Check sheet for the modelled part. Datum: model origin and axes. Units: mm. Coordinates: 2 decimals unless noted, no trailing zeros. Loops run counter-clockwise (first coordinate to the right, second up) from the corner with the lowest first, then second, coordinate; pieces in that order, holes last. Notation, with made-up numbers: (-15.5, 38) -> (0.5, 38) arc R21 cw to (0.5, 57) -> close; hole circle Ø8 at (38, 59). An arc over 180 degrees is marked (long way). Use one line per item in the form item = value.
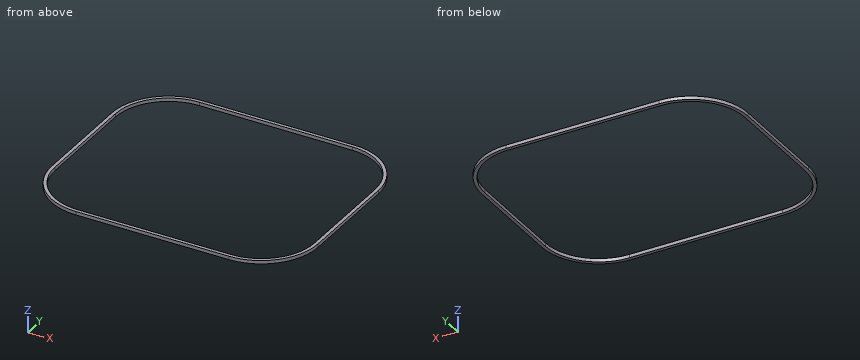
from build123d import *

# Parameters (mm, degrees)
F0_W     = 500
F0_H     = 6.35
F1_DEPTH = 410
F3_DEPTH = 25
F4_W     = 517.022076
F4_H     = 424.169128
F5_DEPTH = 25


with BuildPart() as f1:
    # F0 (on Front) → F1 (new body)
    with BuildSketch(Plane.XZ):
        with Locations((250, 3.175)):
            Rectangle(F0_W, F0_H)
    extrude(amount=F1_DEPTH)

    # F2 (on face) → F3 (cut)
    with BuildSketch(Plane.XY.offset(6.35)):
        with BuildLine():
            Line((393.65, -6.35), (106.35, -6.35))
            ThreePointArc((106.35, -6.35), (35.639322, -35.639322), (6.35, -106.35))
            Line((6.35, -106.35), (6.35, -303.65))
            ThreePointArc((6.35, -303.65), (35.639322, -374.360678), (106.35, -403.65))
            Line((106.35, -403.65), (393.65, -403.65))
            ThreePointArc((393.65, -403.65), (464.360678, -374.360678), (493.65, -303.65))
            Line((493.65, -303.65), (493.65, -106.35))
            ThreePointArc((493.65, -106.35), (464.360678, -35.639322), (393.65, -6.35))
        make_face()
    extrude(amount=-F3_DEPTH, mode=Mode.SUBTRACT)

    # F4 (on face) → F5 (cut)
    with BuildSketch(Plane.XY.offset(6.35)):
        with Locations((249.736218, -205.263791)):
            Rectangle(F4_W, F4_H)
        with BuildLine():
            ThreePointArc((0, -106.35), (31.149194, -31.149194), (106.35, 0))
            Line((106.35, 0), (393.65, 0))
            ThreePointArc((393.65, 0), (468.850806, -31.149194), (500, -106.35))
            Line((500, -106.35), (500, -303.65))
            ThreePointArc((500, -303.65), (468.850806, -378.850806), (393.65, -410))
            Line((393.65, -410), (106.35, -410))
            ThreePointArc((106.35, -410), (31.149194, -378.850806), (0, -303.65))
            Line((0, -303.65), (0, -106.35))
        make_face(mode=Mode.SUBTRACT)
    extrude(amount=-F5_DEPTH, mode=Mode.SUBTRACT)


solid = f1.part
(1) Section check C-C, the plane z = 5. Record the boundary of the cut face in (x, y).
Established:
outline = (0, -303.65) arc R106.35 ccw to (106.35, -410) -> (393.65, -410) arc R106.35 ccw to (500, -303.65) -> (500, -106.35) arc R106.35 ccw to (393.65, 0) -> (106.35, 0) arc R106.35 ccw to (0, -106.35) -> close; hole (6.35, -303.65) arc R100 ccw to (106.35, -403.65) -> (393.65, -403.65) arc R100 ccw to (493.65, -303.65) -> (493.65, -106.35) arc R100 ccw to (393.65, -6.35) -> (106.35, -6.35) arc R100 ccw to (6.35, -106.35) -> close
(2) Section check A-A, the plane y = -245. Record the boundary of the cut face in (x, z), plus the area to 3 significant figures.
Established:
outline = (0, 0) -> (6.35, 0) -> (6.35, 6.35) -> (0, 6.35) -> close; (493.65, 0) -> (500, 0) -> (500, 6.35) -> (493.65, 6.35) -> close
area = 80.6 mm²
(3) Scan lines: line 1 along X through (y, z) = (-308, 5); line 2 along Y through (x, z) = (308, 1.5). Record each from-to range of solid material in increasing order.
Established:
line_1 = 0.09 to 6.44, 493.56 to 499.91
line_2 = -410 to -403.65, -6.35 to 0
(4) Section check B-B, the plane x = 153. Record the boundary of the cut face in (y, z).
Established:
outline = (-410, 0) -> (-403.65, 0) -> (-403.65, 6.35) -> (-410, 6.35) -> close; (-6.35, 0) -> (0, 0) -> (0, 6.35) -> (-6.35, 6.35) -> close
